```python
from build123d import *

# Parameters (mm, degrees)
F0_W     = 15
F0_H     = 25
F1_DEPTH = 3
F2_W     = 10
F2_H     = 10
F3_DEPTH = 2
F4_R     = 3
F6_D     = 3.5


with BuildPart() as f1:
    # F0 (on Top) → F1 (new body)
    with BuildSketch(Plane.XY):
        with Locations((7.5, -12.5)):
            Rectangle(F0_W, F0_H)
    extrude(amount=F1_DEPTH)

    # F2 (on face) → F3 (join)
    with BuildSketch(Plane(origin=(0, 0, 0), x_dir=(1, 0, 0), z_dir=(0, 0, -1))):
        with Locations((5, 5)):
            Rectangle(F2_W, F2_H)
    extrude(amount=F3_DEPTH)

    # F4
    f4_edges = [f1.edges().sort_by_distance(p)[0] for p in [
        (0, 0, 0.5),
        (0, -25, 1.5),
        (15, -25, 1.5),
        (15, 0, 1.5),
    ]]
    fillet(f4_edges, radius=F4_R)

    # F6 (through all)
    with Locations(Plane.XY.offset(3)):
        with Locations((5, -5)):
            Hole(F6_D / 2)


solid = f1.part
```
Input: part model. Units: mm. Frame: model coordinates. A direction names the side the tool comes from. Coordinates: 2 decimals unless noted, no trailing zeros. Write each loop counter-clockwise with the first axis right and the second up, starting at its lowest first coordinate (ties: lowest second). Pieces come first, ordered by that corner, then holes. Notation, with made-up numbers: (42.5, 44.5) -> (65.5, 44.5) arc R14 ccw to (65.5, 54.5) -> close; hole circle Ø8 at (5, 8.5). An arc over 180 degrees is marked (long way). Answer as a JSON object with one key per item and string values.
1. Material intervals for line 1 (Y direction, x = 5, z = 0.9); line 2 (Y direction, x = 5, z = -0.05); line 3 (Z direction, x = 11, y = -0.75), sorted ascending. Write a range as from..to.
Result set:
{"line 1": "y = -25..-6.75, -3.25..0", "line 2": "y = -10..-6.75, -3.25..0", "line 3": "z = 0..3"}
2. Section B-B on x = 5. Return the cut outline in (y, z).
Result set:
{"outline": "(-25, 0) -> (-10, 0) -> (-10, -2) -> (-6.75, -2) -> (-6.75, 3) -> (-25, 3) -> close; (-3.25, -2) -> (0, -2) -> (0, 3) -> (-3.25, 3) -> close"}
3. First-contact query: P1, Ø0.6, axis at x = 5, z = -1, coming from the -Y side; P2, Ø0.6, axis at y = -5, z = -1.5, coming from the +X side; P3, Ø4.5, axis at x = 9.5, y = -11.5, coming from the -Z side. Flat tips, straight axial feed; report the tip coordinate or a pass-through.
Result set:
{"P1": "stops at y = -10", "P2": "stops at x = 10", "P3": "stops at z = -2"}
4. Section A-A on y = -5. Return the cut outline in (x, z), then the cut area to 3 significant figures.
Result set:
{"outline": "(0, -2) -> (3.25, -2) -> (3.25, 3) -> (0, 3) -> close; (6.75, -2) -> (10, -2) -> (10, 0) -> (15, 0) -> (15, 3) -> (6.75, 3) -> close", "area": "47.5 mm2"}
5. Mould query, pull axis X, two halves, no side actions, for faces 1 (the face through (7, -5, -2)), 2 (the face through (15, -13, 1)), 3 (the face through (5.38, -6.71, 0.47)), 4 (the face through (0.86, -24.1, 1.52)). Classes: released by +X, released by -X, zero draft, split by the parting line, or undercut.
Result set:
{"face 1": "zero draft", "face 2": "released by +X", "face 3": "undercut", "face 4": "released by -X"}
6. Section C-C on z = 1.05. Return the cut outline in (x, y).
Result set:
{"outline": "(0, -22) arc R3 ccw to (3, -25) -> (12, -25) arc R3 ccw to (15, -22) -> (15, -3) arc R3 ccw to (12, 0) -> (3, 0) arc R3 ccw to (0, -3) -> close; hole circle Ø3.5 at (5, -5)"}
7. Section D-D on y = -9.25. Return the cut outline in (x, z).
Result set:
{"outline": "(0, -2) -> (10, -2) -> (10, 0) -> (15, 0) -> (15, 3) -> (0, 3) -> close"}
8. Access query for faces 5 (the face through (5, -10, -1)), 6 (the face through (10, -5, -1)), 7 (the face through (7, -25, 1)). Directions: +Z, -Z, +X, -X, +Y, -Y. A direction counts if a zero-diameter tool reaches every point of the face in a straight line with its end or side. Return the directions, or none.
Result set:
{"face 5": "-Z, +X, -X, -Y", "face 6": "-Z, +X, +Y, -Y", "face 7": "+Z, -Z, +X, -X, -Y"}
